```python
from build123d import *

# Parameters (mm, degrees)
BOSS_EXTRUDE1_DEPTH            = 10
SKETCH1_3_W                    = 51
SKETCH1_3_H                    = 28.56
BOSS_EXTRUDE2_DEPTH            = 5
CUT_EXTRUDE1_REACH             = 79.48
SKETCH3_R                      = 3
SKETCH3_R_2                    = 2
CUT_EXTRUDE1_DIRECTION_2_REACH = 79.48
BOSS_EXTRUDE3_DEPTH            = 12.5
BOSS_EXTRUDE3_DEPTH_BACK       = 12.5
SKETCH3_5_R                    = 3
SKETCH3_5_R_2                  = 2
CUT_EXTRUDE5_DEPTH             = 10.5
CUT_EXTRUDE5_DEPTH_BACK        = 10.5
SKETCH3_12_R                   = 3
SKETCH3_12_R_2                 = 2
FILLET1_R                      = 10


with BuildPart() as part:
    # Sketch1 → Boss-Extrude1 (new body)
    # profile 1 of 3: a face of its own
    with BuildSketch(Plane(origin=(0, 0, 0), x_dir=(1, 0, 0), z_dir=(0, 1, 0))):
        Polygon((-30.5, 47.36), (-30.5, 15.5), (-25.5, 15.5), (-25.5, 44.06), (25.5, 44.06), (25.5, 15.5), (30.5, 15.5), (30.5, 47.36), align=None)
    # profile 2 of 3: a face of its own
    with BuildSketch(Plane(origin=(0, 0, 0), x_dir=(1, 0, 0), z_dir=(0, 1, 0))):
        Polygon((30.5, 15.5), (-30.5, 15.5), (-60.5, 15.5), (-60.5, -15.5), (-30.5, -15.5), (30.5, -15.5), (60.5, -15.5), (60.5, 15.5), align=None)
        Polygon((30.5, 10.5), (-30.5, 10.5), (-55.5, 10.5), (-55.5, -10.5), (-30.5, -10.5), (30.5, -10.5), (55.5, -10.5), (55.5, 10.5), align=None, mode=Mode.SUBTRACT)
    # profile 3 of 3: a face of its own
    with BuildSketch(Plane(origin=(0, 0, 0), x_dir=(1, 0, 0), z_dir=(0, 1, 0))):
        Polygon((-30.5, -15.5), (-30.5, -47.36), (30.5, -47.36), (30.5, -15.5), (25.5, -15.5), (25.5, -44.06), (-25.5, -44.06), (-25.5, -15.5), align=None)
    extrude(amount=BOSS_EXTRUDE1_DEPTH)

    # Sketch1<3> → Boss-Extrude2 (add)
    # profile 1 of 5: a face of its own
    with BuildSketch(Plane(origin=(0, 0, 0), x_dir=(1, 0, 0), z_dir=(0, 1, 0))):
        Polygon((-30.5, -15.5), (-30.5, -47.36), (30.5, -47.36), (30.5, -15.5), (25.5, -15.5), (25.5, -44.06), (-25.5, -44.06), (-25.5, -15.5), align=None)
    # profile 2 of 5: a face of its own
    with BuildSketch(Plane(origin=(0, 0, 0), x_dir=(1, 0, 0), z_dir=(0, 1, 0))):
        Polygon((-60.5, -15.5), (-30.5, -15.5), (-25.5, -15.5), (25.5, -15.5), (30.5, -15.5), (60.5, -15.5), (60.5, 15.5), (30.5, 15.5), (25.5, 15.5), (-25.5, 15.5), (-30.5, 15.5), (-60.5, 15.5), align=None)
        Polygon((-55.5, 10.5), (-30.5, 10.5), (30.5, 10.5), (55.5, 10.5), (55.5, -10.5), (30.5, -10.5), (-30.5, -10.5), (-55.5, -10.5), align=None, mode=Mode.SUBTRACT)
    # profile 3 of 5: a face of its own
    with BuildSketch(Plane(origin=(0, 0, 0), x_dir=(1, 0, 0), z_dir=(0, 1, 0))):
        with Locations((0, -29.78)):
            Rectangle(SKETCH1_3_W, SKETCH1_3_H)
        with BuildLine():
            ThreePointArc((-15.5, -27.73), (-20.59, -22.64), (-15.5, -17.55))
            Line((-15.5, -17.55), (15.5, -17.55))
            ThreePointArc((15.5, -17.55), (20.59, -22.64), (15.5, -27.73))
            Line((15.5, -27.73), (-15.5, -27.73))
        make_face(mode=Mode.SUBTRACT)
        with BuildLine():
            Line((15.5, -42.01), (-15.5, -42.01))
            ThreePointArc((-15.5, -42.01), (-20.59, -36.92), (-15.5, -31.83))
            Line((-15.5, -31.83), (15.5, -31.83))
            ThreePointArc((15.5, -31.83), (20.59, -36.92), (15.5, -42.01))
        make_face(mode=Mode.SUBTRACT)
    # profile 4 of 5: a face of its own
    with BuildSketch(Plane(origin=(0, 0, 0), x_dir=(1, 0, 0), z_dir=(0, 1, 0))):
        Polygon((-30.5, 47.36), (-30.5, 15.5), (-25.5, 15.5), (-25.5, 44.06), (25.5, 44.06), (25.5, 15.5), (30.5, 15.5), (30.5, 47.36), align=None)
    # profile 5 of 5: a face of its own
    with BuildSketch(Plane(origin=(0, 0, 0), x_dir=(1, 0, 0), z_dir=(0, 1, 0))):
        with Locations((0, 29.78)):
            Rectangle(SKETCH1_3_W, SKETCH1_3_H)
        with BuildLine():
            Line((15.5, 17.55), (-15.5, 17.55))
            ThreePointArc((-15.5, 17.55), (-20.59, 22.64), (-15.5, 27.73))
            Line((-15.5, 27.73), (15.5, 27.73))
            ThreePointArc((15.5, 27.73), (20.59, 22.64), (15.5, 17.55))
        make_face(mode=Mode.SUBTRACT)
        with BuildLine():
            ThreePointArc((-15.5, 31.83), (-20.59, 36.92), (-15.5, 42.01))
            Line((-15.5, 42.01), (15.5, 42.01))
            ThreePointArc((15.5, 42.01), (20.59, 36.92), (15.5, 31.83))
            Line((15.5, 31.83), (-15.5, 31.83))
        make_face(mode=Mode.SUBTRACT)
    extrude(amount=-BOSS_EXTRUDE2_DEPTH)

    # Cut-Extrude1: up to this face of the body (flat: up to its plane)
    cut_extrude1_end = Plane(part.part.faces().sort_by_distance((-45.5, 2.5, -15.5))[0])
    # Sketch3 → Cut-Extrude1 (cut, up to the picked face)
    with BuildSketch(Plane.XY, mode=Mode.PRIVATE) as cut_extrude1_sk1:
        with Locations((-46.5, 1)):
            Circle(SKETCH3_R)
        with Locations((-46.5, 1)):
            Circle(SKETCH3_R_2, mode=Mode.SUBTRACT)
    cut_extrude1_tool1 = split(extrude(cut_extrude1_sk1.sketch, amount=-CUT_EXTRUDE1_REACH, mode=Mode.PRIVATE), bisect_by=cut_extrude1_end, keep=Keep.BOTH, mode=Mode.PRIVATE)
    # Sketch3 → Cut-Extrude1 (cut, up to the picked face)
    with BuildSketch(Plane.XY, mode=Mode.PRIVATE) as cut_extrude1_sk2:
        with Locations((-46.5, 1)):
            Circle(SKETCH3_R_2)
    cut_extrude1_tool2 = split(extrude(cut_extrude1_sk2.sketch, amount=-CUT_EXTRUDE1_REACH, mode=Mode.PRIVATE), bisect_by=cut_extrude1_end, keep=Keep.BOTH, mode=Mode.PRIVATE)
    # Sketch3 → Cut-Extrude1 (cut, up to the picked face)
    with BuildSketch(Plane.XY, mode=Mode.PRIVATE) as cut_extrude1_sk3:
        with Locations((46.5, 1)):
            Circle(SKETCH3_R)
        with Locations((46.5, 1)):
            Circle(SKETCH3_R_2, mode=Mode.SUBTRACT)
    cut_extrude1_tool3 = split(extrude(cut_extrude1_sk3.sketch, amount=-CUT_EXTRUDE1_REACH, mode=Mode.PRIVATE), bisect_by=cut_extrude1_end, keep=Keep.BOTH, mode=Mode.PRIVATE)
    # Sketch3 → Cut-Extrude1 (cut, up to the picked face)
    with BuildSketch(Plane.XY, mode=Mode.PRIVATE) as cut_extrude1_sk4:
        with Locations((46.5, 1)):
            Circle(SKETCH3_R_2)
    cut_extrude1_tool4 = split(extrude(cut_extrude1_sk4.sketch, amount=-CUT_EXTRUDE1_REACH, mode=Mode.PRIVATE), bisect_by=cut_extrude1_end, keep=Keep.BOTH, mode=Mode.PRIVATE)
    add(cut_extrude1_tool1.solids().sort_by(Axis((-49.415147, 1, 0), (0, 0, -1)))[0], mode=Mode.SUBTRACT)
    add(cut_extrude1_tool2.solids().sort_by(Axis((-46.5, 1, 0), (0, 0, -1)))[0], mode=Mode.SUBTRACT)
    add(cut_extrude1_tool3.solids().sort_by(Axis((43.584853, 1, 0), (0, 0, -1)))[0], mode=Mode.SUBTRACT)
    add(cut_extrude1_tool4.solids().sort_by(Axis((46.5, 1, 0), (0, 0, -1)))[0], mode=Mode.SUBTRACT)

    # Cut-Extrude1 direction 2: up to this face of the body (flat: up to its plane)
    cut_extrude1_direction_2_end = Plane(part.part.faces().sort_by_distance((-45.5, 2.5, 15.5))[0])
    # Sketch3 → Cut-Extrude1 direction 2 (cut, up to the picked face)
    with BuildSketch(Plane.XY, mode=Mode.PRIVATE) as cut_extrude1_direction_2_sk1:
        with Locations((-46.5, 1)):
            Circle(SKETCH3_R)
        with Locations((-46.5, 1)):
            Circle(SKETCH3_R_2, mode=Mode.SUBTRACT)
    cut_extrude1_direction_2_tool1 = split(extrude(cut_extrude1_direction_2_sk1.sketch, amount=CUT_EXTRUDE1_DIRECTION_2_REACH, mode=Mode.PRIVATE), bisect_by=cut_extrude1_direction_2_end, keep=Keep.BOTH, mode=Mode.PRIVATE)
    # Sketch3 → Cut-Extrude1 direction 2 (cut, up to the picked face)
    with BuildSketch(Plane.XY, mode=Mode.PRIVATE) as cut_extrude1_direction_2_sk2:
        with Locations((-46.5, 1)):
            Circle(SKETCH3_R_2)
    cut_extrude1_direction_2_tool2 = split(extrude(cut_extrude1_direction_2_sk2.sketch, amount=CUT_EXTRUDE1_DIRECTION_2_REACH, mode=Mode.PRIVATE), bisect_by=cut_extrude1_direction_2_end, keep=Keep.BOTH, mode=Mode.PRIVATE)
    # Sketch3 → Cut-Extrude1 direction 2 (cut, up to the picked face)
    with BuildSketch(Plane.XY, mode=Mode.PRIVATE) as cut_extrude1_direction_2_sk3:
        with Locations((46.5, 1)):
            Circle(SKETCH3_R)
        with Locations((46.5, 1)):
            Circle(SKETCH3_R_2, mode=Mode.SUBTRACT)
    cut_extrude1_direction_2_tool3 = split(extrude(cut_extrude1_direction_2_sk3.sketch, amount=CUT_EXTRUDE1_DIRECTION_2_REACH, mode=Mode.PRIVATE), bisect_by=cut_extrude1_direction_2_end, keep=Keep.BOTH, mode=Mode.PRIVATE)
    # Sketch3 → Cut-Extrude1 direction 2 (cut, up to the picked face)
    with BuildSketch(Plane.XY, mode=Mode.PRIVATE) as cut_extrude1_direction_2_sk4:
        with Locations((46.5, 1)):
            Circle(SKETCH3_R_2)
    cut_extrude1_direction_2_tool4 = split(extrude(cut_extrude1_direction_2_sk4.sketch, amount=CUT_EXTRUDE1_DIRECTION_2_REACH, mode=Mode.PRIVATE), bisect_by=cut_extrude1_direction_2_end, keep=Keep.BOTH, mode=Mode.PRIVATE)
    add(cut_extrude1_direction_2_tool1.solids().sort_by(Axis((-49.415147, 1, 0), (0, 0, 1)))[0], mode=Mode.SUBTRACT)
    add(cut_extrude1_direction_2_tool2.solids().sort_by(Axis((-46.5, 1, 0), (0, 0, 1)))[0], mode=Mode.SUBTRACT)
    add(cut_extrude1_direction_2_tool3.solids().sort_by(Axis((43.584853, 1, 0), (0, 0, 1)))[0], mode=Mode.SUBTRACT)
    add(cut_extrude1_direction_2_tool4.solids().sort_by(Axis((46.5, 1, 0), (0, 0, 1)))[0], mode=Mode.SUBTRACT)

    # Sketch3<5> → Boss-Extrude3 (add, two sides: drawn at the far end of the back side and taken through both)
    # profile 1 of 2: a face of its own
    with BuildSketch(Plane.XY.offset(-BOSS_EXTRUDE3_DEPTH_BACK)):
        with Locations((-46.5, 1)):
            Circle(SKETCH3_5_R)
        with Locations((-46.5, 1)):
            Circle(SKETCH3_5_R_2, mode=Mode.SUBTRACT)
    # profile 2 of 2: a face of its own
    with BuildSketch(Plane.XY.offset(-BOSS_EXTRUDE3_DEPTH_BACK)):
        with Locations((46.5, 1)):
            Circle(SKETCH3_5_R)
        with Locations((46.5, 1)):
            Circle(SKETCH3_5_R_2, mode=Mode.SUBTRACT)
    extrude(amount=BOSS_EXTRUDE3_DEPTH + BOSS_EXTRUDE3_DEPTH_BACK)

    # Sketch3<12> → Cut-Extrude5 (cut, two sides: drawn at the far end of the back side and taken through both)
    # profile 1 of 2: a face of its own
    with BuildSketch(Plane.XY.offset(-CUT_EXTRUDE5_DEPTH_BACK)):
        with Locations((46.5, 1)):
            Circle(SKETCH3_12_R)
        with Locations((46.5, 1)):
            Circle(SKETCH3_12_R_2, mode=Mode.SUBTRACT)
    # profile 2 of 2: a face of its own
    with BuildSketch(Plane.XY.offset(-CUT_EXTRUDE5_DEPTH_BACK)):
        with Locations((-46.5, 1)):
            Circle(SKETCH3_12_R)
        with Locations((-46.5, 1)):
            Circle(SKETCH3_12_R_2, mode=Mode.SUBTRACT)
    extrude(amount=CUT_EXTRUDE5_DEPTH + CUT_EXTRUDE5_DEPTH_BACK, mode=Mode.SUBTRACT)

    # Fillet1
    fillet1_edges = [part.edges().sort_by_distance(p)[0] for p in [
        (60.5, 2.5, -15.5),
        (60.5, 2.5, 15.5),
        (30.5, 2.5, 47.36),
        (-30.5, 2.5, 47.36),
        (-60.5, 2.5, 15.5),
        (-60.5, 2.5, -15.5),
        (-30.5, 2.5, -47.36),
        (30.5, 2.5, -47.36),
    ]]
    fillet(fillet1_edges, radius=FILLET1_R)


solid = part.part
```
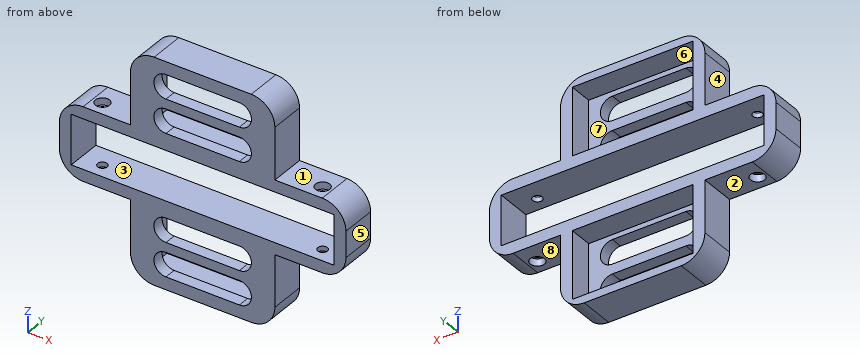
Geometry: final body of the model. Coordinates: model frame, mm. Face numbers are marked on the shaded views. A direction names the side the tool comes from. Coordinates: 2 decimals unless noted, no trailing zeros. Loops run counter-clockwise (first coordinate to the right, second up) from the corner with the lowest first, then second, coordinate; pieces in that order, holes last. Notation, with made-up numbers: (36.5, -27) -> (80.5, -27) arc R19 ccw to (80.5, -18) -> close; hole circle Ø5 at (-37, 86). An arc over 180 degrees is marked (long way). Use a Markdown table: item, result. Add a question column.
(1) Section query B-B, the plane z = 22.64. Return loops of the section in (x, y), plus the area to 3 significant figures.
(2) Access query for the marked faces 1, 2, 3 and 4. Directions: +Z, -Z, +X, -X, +Y, -Y. A direction counts if a zero-diameter tool reaches every point of the face in a straight line with its end or side. Return the directions, or none.
(3) Section query A-A, the plane x = 46.5. Return loops of the section in (y, z).
(4) Mould query, pull axis X, two halves, no side actions, for the marked faces 5, 6, 7 and 8. Classes: pulls with the +X half, pulls with the -X half, needs draft (parallel to the pull), parting line crosses it, or undercut.
(5) Pin query (flat end, axial travel): pin 1 Ø2 at (x, z) = (4.5, -25) entering from +Y; pin 2 Ø3 at (x, y) = (-47.5, 2) entering from -Z; pin 3 Ø8 at (x, y) = (46.5, 1) entering from -Z; pin 4 Ø3 at (x, y) = (45, -0.5) entering from +Z. Return the tip coordinate at first contact, or that it passes through.
(6) Line query: line 1 along Z through (x, y) = (8, 8.25); line 2 along Z through (x, y) = (4, -0.5); line 3 along Z through (x, y) = (46.5, -4). Output: solid intervals per line, ascending.
(7) Section query C-C, the plane y = 6. State how many separate pieces and enclosed holes the cut face has, plus the area to 3 significant figures.
Answer:
| question | item | result |
|---|---|---|
| 1 | outline | (-30.5, -5) -> (-20.59, -5) -> (-20.59, 0) -> (-25.5, 0) -> (-25.5, 10) -> (-30.5, 10) -> close; (20.59, -5) -> (30.5, -5) -> (30.5, 10) -> (25.5, 10) -> (25.5, 0) -> (20.59, 0) -> close |
| 1 | area | 199 mm^2 |
| 2 | face 1 | +Z, +X, +Y, -Y |
| 2 | face 2 | -Z, -X, +Y, -Y |
| 2 | face 3 | +Y, -Y |
| 2 | face 4 | +Z, -X, +Y, -Y |
| 3 | outline | (-5, -15.5) -> (-2, -15.5) -> (-2, -12.5) -> (-1, -12.5) -> (-1, -10.5) -> (-5, -10.5) -> close; (-5, 10.5) -> (-1, 10.5) -> (-1, 12.5) -> (-2, 12.5) -> (-2, 15.5) -> (-5, 15.5) -> close; (3, -12.5) -> (4, -12.5) -> (4, -15.5) -> (10, -15.5) -> (10, -10.5) -> (3, -10.5) -> close; (3, 10.5) -> (10, 10.5) -> (10, 15.5) -> (4, 15.5) -> (4, 12.5) -> (3, 12.5) -> close |
| 4 | face 5 | pulls with the +X half |
| 4 | face 6 | undercut |
| 4 | face 7 | undercut |
| 4 | face 8 | needs draft |
| 5 | pin 1 | passes through |
| 5 | pin 2 | stops at z = -12.5 |
| 5 | pin 3 | stops at z = -15.5 |
| 5 | pin 4 | stops at z = 15.5 |
| 6 | line 1 | z = -47.36 to -44.06, -15.5 to -10.5, 10.5 to 15.5, 44.06 to 47.36 |
| 6 | line 2 | z = -47.36 to -42.01, -31.83 to -27.73, -17.55 to -10.5, 10.5 to 17.55, 27.73 to 31.83, 42.01 to 47.36 |
| 6 | line 3 | z = -15.5 to -10.5, 10.5 to 15.5 |
| 7 | separate pieces | 1 |
| 7 | enclosed holes | 3 |
| 7 | area | 2,220 mm^2 |
